Geometry: final body of the model. Coordinates: model frame, mm. Face numbers are marked on the shaded views. A direction names the side the tool comes from. Give positions to 0.01 mm unless a question says otherwise; leave off trailing zeros. Write item = value, one per line.
```python
from build123d import *

# Parameters (mm, degrees)
ESQUISSE2_R                  = 14.25
BOSS_EXTRU_1_DEPTH           = 3.25
ESQUISSE3_R                  = 1.2
ENL_V_MAT_EXTRU_1_DEPTH      = 4.25
ESQUISSE10_R                 = 1.7
ENL_V_MAT_EXTRU_2_DEPTH      = 1
ENL_V_MAT_EXTRU_2_DEPTH_BACK = 7.5
ESQUISSE17_R                 = 4
ENL_V_MAT_EXTRU_8_DEPTH      = 7.5
ESQUISSE13_R                 = 1.4
ENL_V_MAT_EXTRU_4_DEPTH      = 35.402543264
ESQUISSE20_R                 = 2.5
ENL_V_MAT_EXTRU_9_DEPTH      = 3


with BuildPart() as part:
    # Esquisse2 → Boss.-Extru.1 (new body, symmetric)
    with BuildSketch(Plane.XY):
        Circle(ESQUISSE2_R)
    extrude(amount=BOSS_EXTRU_1_DEPTH, both=True)

    # Esquisse3 → Enlèv. mat.-Extru.1 (cut, through all)
    with BuildSketch(Plane.XY):
        with Locations((0, 8.25)):
            Circle(ESQUISSE3_R)
        with Locations((-8.25, 0)):
            Circle(ESQUISSE3_R)
        with Locations((0, -8.25)):
            Circle(ESQUISSE3_R)
        with Locations((8.25, 0)):
            Circle(ESQUISSE3_R)
    extrude(amount=ENL_V_MAT_EXTRU_1_DEPTH, mode=Mode.SUBTRACT)

    # Esquisse10 → Enlèv. mat.-Extru.2 (cut, two sides)
    with BuildSketch(Plane(origin=(0, 0, -3.25), x_dir=(-1, 0, 0), z_dir=(0, 0, -1))) as enl_v_mat_extru_2_sk:
        with Locations((-8.25, 0)):
            Circle(ESQUISSE10_R)
        with Locations((0, 8.25)):
            Circle(ESQUISSE10_R)
        with Locations((8.25, 0)):
            Circle(ESQUISSE10_R)
        with Locations((0, -8.25)):
            Circle(ESQUISSE10_R)
    extrude(amount=ENL_V_MAT_EXTRU_2_DEPTH, mode=Mode.SUBTRACT)
    extrude(enl_v_mat_extru_2_sk.sketch, amount=-ENL_V_MAT_EXTRU_2_DEPTH_BACK, mode=Mode.SUBTRACT)

    # Esquisse17 → Enlèv. mat.-Extru.8 (cut, through all)
    with BuildSketch(Plane.XY.offset(3.25)):
        Circle(ESQUISSE17_R)
    extrude(amount=-ENL_V_MAT_EXTRU_8_DEPTH, mode=Mode.SUBTRACT)

    # Esquisse13 → Enlèv. mat.-Extru.4 (cut, through all)
    with BuildSketch(Plane(origin=(10.076271632, -10.076271632, 0), x_dir=(-0.707106781, -0.707106781, 0), z_dir=(0.707106781, -0.707106781, 0))):
        Circle(ESQUISSE13_R)
    extrude(amount=-ENL_V_MAT_EXTRU_4_DEPTH, mode=Mode.SUBTRACT)

    # Esquisse18 → Enlèvement de matière-Révolution1 (revolve, cut)
    with BuildSketch(Plane(origin=(0, 0, 0), x_dir=(1, 0, 0), z_dir=(0, 1, 0))):
        Polygon((14.25, 2.5), (12.152250922, 0), (14.25, -2.5), align=None)
    revolve(axis=Axis((0, 0, -3.25), (0, 0, 1)), mode=Mode.SUBTRACT)

    # Esquisse20 → Enlèv. mat.-Extru.9 (cut)
    with BuildSketch(Plane.XY.offset(3.25)):
        with Locations((0, 8.25)):
            Circle(ESQUISSE20_R)
        with Locations((8.25, 0)):
            Circle(ESQUISSE20_R)
        with Locations((-8.25, 0)):
            Circle(ESQUISSE20_R)
        with Locations((0, -8.25)):
            Circle(ESQUISSE20_R)
    extrude(amount=-ENL_V_MAT_EXTRU_9_DEPTH, mode=Mode.SUBTRACT)


solid = part.part
```
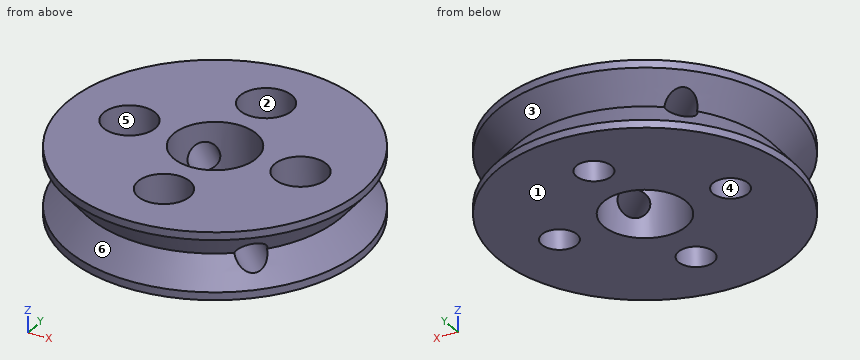
1) Line query: line 1 (Y direction, x = -1.25, z = 1); line 2 (Y direction, x = 0, z = -0.5); line 3 (Z direction, x = 1.25, y = 7). Output: solid intervals per line, ascending. Write a range as from..to.
Check sheet entries:
line_1 = -12.93..-10.42, -6.08..-3.8, 3.8..6.08, 10.42..12.93
line_2 = -12.57..-9.95, -6.55..-4, 4..6.55, 9.95..12.57
line_3 = -3.25..0.25
2) Section query B-B (y = 0). Count the separate pieces of the cut face and the enclosed holes in it, plus the area to 3 significant figures.
Check sheet entries:
separate_pieces = 4
enclosed_holes = 0
area = 69.0 mm²
3) First-contact query: P1, Ø3, axis at y = 8, z = -2, coming from the -X side; P2, Ø3, axis at x = 8.5, z = 0.5, coming from the +Y side; P3, Ø4, axis at x = 0, y = 8.25, coming from the +Z side. Flat tips, straight axial feed; report the tip coordinate or a pass-through.
Check sheet entries:
P1 = -12.64
P2 = 11.26
P3 = 0.25
4) Reachability of the marked faces 4, 5 and 6 from +Z, -Z, +X, -X, +Y, -Y: full face, straight path, thin tool, end or side. Return the list, or none.
Check sheet entries:
face_4 = +Z, -Z
face_5 = +Z
face_6 = none
5) Mould query, pull axis X, two halves, no side actions, for the marked faces 1, 2 and 3. Classes: +X half, -X half, draft (parallel to the pull), parting line (faces both ways), or undercut.
Check sheet entries:
face_1 = draft
face_2 = undercut
face_3 = parting line
